Model file for the job. Use its own axes, mm. Face numbers are marked on the shaded views. A direction names the side the tool comes from. Coordinates: 2 decimals unless noted, no trailing zeros. Order: outer loops, then holes, each group sorted by start corner. A loop starts at its lowest first (then second) coordinate and runs counter-clockwise, first axis right, second up. Notation, with made-up numbers: (-36.75, -16.75) -> (-31.75, -16.75) arc R11 ccw to (-31.75, -12.75) -> close; hole circle Ø2 at (-31, -39.5). An arc over 180 degrees is marked (long way). Write item = value, one per line. Start each with the question number.
Q1. Wall check: line 1 (X direction, y = 6, z = -6); line 2 (Y direction, x = 12.4, z = 0); line 3 (Z direction, x = 12.6, y = 0). Give the ranges that are in metal, low to high. Write a range as from..to.
Q2. Cut at C-C, the plane z = -1. List the corners of the cut face in (x, y), plus the area to 3 significant figures.
Q3. 3-axis set-ups, long thin cutter, end or side, ignore diameter. For the marked faces 1, 2 and 3: which of +Z, -Z, +X, -X, +Y, -Y reach the whole face in a straight line?
Q4. Mould opens along Z. For the marked faces 4, 5, 6 and 7 say: +Z half, -Z half, draft (parallel to the pull), parting line (faces both ways), or undercut.
Q5. Cut at A-A, the plane x = 12.5. List the corners of the cut face in (y, z), plus the area to 3 significant figures.
Q6. Flat gauge pins, fed straight in: pin 1 (6.5 mm diameter, centred on x = 6.5, z = 0, fed in from +Y); pin 2 (4 mm diameter, centred on x = 12.5, y = -11.5, fed in from +Z); pin 3 (6.5 mm diameter, centred on x = 6, z = 1.5, fed in from +Y); pin 4 (1.5 mm diameter, centred on x = 2, z = 8.5, fed in from +Y). Where does each tip first touch, or does it go through?
Q7. Cut at D-D, the plane x = 7. List the corners of the cut face in (y, z), plus the area to 3 significant figures.
Q8. Cut at B-B, the plane y = 0. List the corners of the cut face in (x, z).
from build123d import *
from OCP.BRepFilletAPI import BRepFilletAPI_MakeChamfer

# Parameters (mm, degrees)
SKETCH9_R           = 2
BOSS_EXTRUDE3_DEPTH = 14
SKETCH10_R          = 2
CUT_EXTRUDE7_DEPTH  = 14
SKETCH11_W          = 8
SKETCH11_H          = 26.663957413
CUT_EXTRUDE8_DEPTH  = 25
FILLET1_R           = 2
CHAMFER1_SIZE       = 2.5
CHAMFER1_SIZE2      = 4.365846821
CHAMFER1_SIZE2_2    = 4.330127019


with BuildPart() as part:
    # Sketch9 → Boss-Extrude3 (new body)
    with BuildSketch(Plane(origin=(0, 0, 0), x_dir=(0, 0, -1), z_dir=(1, 0, 0))):
        with BuildLine():
            Line((8, 5.053889445), (8, -49.642014822))
            Line((8, -49.642014822), (-8, -49.642014822))
            Line((-8, -49.642014822), (-8, -10.875806049))
            ThreePointArc((-8, -10.875806049), (-8.427714838, -7.982476346), (-9.674271354, -5.336650652))
            ThreePointArc((-9.674271354, -5.336650652), (-7.418447874, 8.870328147), (6.925281884, 7.78202542))
            ThreePointArc((6.925281884, 7.78202542), (7.721634556, 6.519985019), (8, 5.053889445))
        make_face()
        Circle(SKETCH9_R, mode=Mode.SUBTRACT)
        with BuildLine():
            Line((5.5, -41.5), (5.5, -25.762364524))
            ThreePointArc((5.5, -25.762364524), (3.987567872, -22.111030369), (0.336233717, -20.598598241))
            Line((0.336233717, -20.598598241), (-0.410415455, -20.598598241))
            ThreePointArc((-0.410415455, -20.598598241), (-4.070351606, -22.119652678), (-5.574124284, -25.786723302))
            Line((-5.574124284, -25.786723302), (-5.5, -41.5))
            Line((-5.5, -41.5), (5.5, -41.5))
        make_face(mode=Mode.SUBTRACT)
    extrude(amount=BOSS_EXTRUDE3_DEPTH)

    # Sketch10 → Cut-Extrude7 (cut)
    with BuildSketch(Plane.XZ.offset(49.642014822)):
        with Locations(Location((7, 0, 0), (0, 0, 270))):
            Circle(SKETCH10_R)
    extrude(amount=-CUT_EXTRUDE7_DEPTH, mode=Mode.SUBTRACT)

    # Sketch11 → Cut-Extrude8 (cut)
    with BuildSketch(Plane(origin=(0, 16, 0), x_dir=(1, 0, 0), z_dir=(0, 1, 0))):
        with Locations((7, -2.726740944)):
            Rectangle(SKETCH11_W, SKETCH11_H)
    extrude(amount=-CUT_EXTRUDE8_DEPTH, mode=Mode.SUBTRACT)

    # Fillet1
    fillet1_edges = [part.edges().sort_by_distance(p)[0] for p in [
        (7, -49.642014822, 8),
        (7, -49.642014822, -8),
    ]]
    fillet(fillet1_edges, radius=FILLET1_R)

    # Chamfer1: one chamfer whose edges measure the first distance from different faces: ONE call of the kernel's chamfer builder (chamfer() names one face for all edges)
    chamfer1_edges_1 = [part.edges().sort_by_distance(p)[0] for p in [
        (7, -41.5, 5.5),
    ]]
    chamfer1_side_1 = [part.faces().sort_by_distance(p)[0] for p in [
        (7, -41.5, 5.321955062),
    ]]
    chamfer1_edges_2 = [part.edges().sort_by_distance(p)[0] for p in [
        (7, -41.5, -5.5),
    ]]
    chamfer1_side_2 = [part.faces().sort_by_distance(p)[0] for p in [
        (7, -41.5, 5.321955062),
    ]]
    chamfer1 = BRepFilletAPI_MakeChamfer(part.part.solid().wrapped)
    for e in chamfer1_edges_1:
        chamfer1.Add(CHAMFER1_SIZE, CHAMFER1_SIZE2, e.wrapped, chamfer1_side_1[0].wrapped)  # the first distance lies on this face
    for e in chamfer1_edges_2:
        chamfer1.Add(CHAMFER1_SIZE, CHAMFER1_SIZE2_2, e.wrapped, chamfer1_side_2[0].wrapped)  # the first distance lies on this face
    add(Compound.cast(chamfer1.Shape()), mode=Mode.REPLACE)


solid = part.part
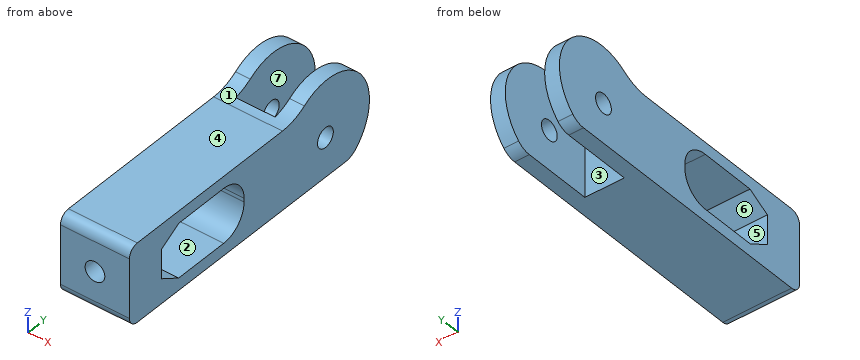
Here are the results:
q1.line_1 = 0..3, 11..14
q1.line_2 = -49.64..-41.5, -20.6..-2, 2..11.12
q1.line_3 = -8..-2, 2..11.44
q2.outline = (0, -49.64) -> (5.27, -49.64) -> (5.27, -41.5) -> (0, -41.5) -> close; (0, -20.64) -> (14, -20.64) -> (14, -1.73) -> (11, -1.73) -> (11, -9) -> (3, -9) -> (3, -1.73) -> (0, -1.73) -> close; (0, 1.73) -> (3, 1.73) -> (3, 11) -> (0, 11) -> close; (8.73, -49.64) -> (14, -49.64) -> (14, -41.5) -> (8.73, -41.5) -> close; (11, 1.73) -> (14, 1.73) -> (14, 11) -> (11, 11) -> close
q2.area = 348 mm²
q3.face_1 = +Z, +X, -X, -Y
q3.face_2 = +X, -X
q3.face_3 = +Z, -Z, +Y
q4.face_4 = +Z half
q4.face_5 = undercut
q4.face_6 = undercut
q4.face_7 = draft
q5.outline = (-49.64, -6) arc R2 ccw to (-47.64, -8) -> (5.05, -8) arc R4 ccw to (7.78, -6.93) arc R10.61 ccw to (-5.34, 9.67) arc R10 cw to (-10.88, 8) -> (-47.64, 8) arc R2 ccw to (-49.64, 6) -> close; hole (-41.5, -3) -> (-37.17, -5.5) -> (-25.76, -5.5) arc R5.16 ccw to (-20.6, -0.34) -> (-20.6, 0.41) arc R5.16 ccw to (-25.79, 5.57) -> (-37.13, 5.52) -> (-41.5, 3) -> close; hole circle Ø4 at (0, 0)
q5.area = 770 mm²
q6.pin_1 = -9
q6.pin_2 = 8.1
q6.pin_3 = 11.16
q6.pin_4 = 8.6
q7.outline = (-49.64, -6) arc R2 ccw to (-47.64, -8) -> (-9, -8) -> (-9, 8.18) arc R10 cw to (-10.88, 8) -> (-47.64, 8) arc R2 ccw to (-49.64, 6) -> (-49.64, 2) -> (-41.5, 2) -> (-41.5, 3) -> (-37.13, 5.52) -> (-25.79, 5.57) arc R5.16 cw to (-20.6, 0.41) -> (-20.6, -0.34) arc R5.16 cw to (-25.76, -5.5) -> (-37.17, -5.5) -> (-41.5, -3) -> (-41.5, -2) -> (-49.64, -2) -> close
q7.area = 408 mm²
q8.outline = (0, -8) -> (3, -8) -> (3, -2) -> (0, -2) -> close; (0, 2) -> (3, 2) -> (3, 11.44) -> (0, 11.44) -> close; (11, -8) -> (14, -8) -> (14, -2) -> (11, -2) -> close; (11, 2) -> (14, 2) -> (14, 11.44) -> (11, 11.44) -> close
